Autodesk Inventor part; units mm, degrees
ref_plane "Work Plane1" through (44.45, -80.8985, 0) normal (0, -1, 0) x (1, 0, 0)
ref_plane "YZ Plane" through (0, 0, 0) normal (1, 0, 0) x (0, 1, 0)
ref_plane "XZ Plane" through (0, 0, 0) normal (0, 1, 0) x (-1, 0, 0)
sketch "Sketch1" plane through (0, 0, 0) normal (0, 0, 1) x (1, 0, 0)
  line L0 (0, 0) -> (88.9, 0)
  line L1 (0, 0) -> (-0.8653, 0)
  line L2 (88.9, 0) -> (18.4478, 0)
  line L3 (88.9, 22.8434) -> (88.9, 0)
  line L4 (0, 0) -> (-3, 0)
  line L5 (-3, 0) -> (-3, 76.2)
  line L6 (-3, 76.2) -> (0, 76.2)
  line L7 (0, 76.2) -> (0, 0)
  line L8 (88.9, 0) -> (91.9, 0)
  line L9 (91.9, 0) -> (91.9, 76.2)
  line L10 (91.9, 76.2) -> (88.9, 76.2)
  line L11 (88.9, 76.2) -> (88.9, 0)
  arc A0 (88.9, 76.2) -> (0, 76.2) centre (44.45, 1.8166) ccw
  arc A1 (91.9, 76.2) -> (-3, 76.2) centre (44.45, 4.8166) ccw
  dimension "d8" = 3
  dimension "d9" = 76.2
  dimension "d10" = 88.9
  dimension "d11" = 3
  dimension "d12" = 3
extrude "Extrusion1" add sketch "Sketch1" along normal blind 12.6 contours L1 L4 L5 L6 L7 | L6 A1 L10 A0 | L3 L11 L10 L9 L8
sketch "Sketch2" plane through (91.9, 0, 0) normal (1, 0, 0) x (0, 0, -1)
  line L0 (0, 0) -> (-6.3, 0)
  line L1 (-6.3, 0) -> (-6.3, 30)
  line L2 (-6.3, 30) -> (0, 30)
  line L3 (0, 30) -> (0, 0)
  circle A0 centre (-6.3, 30) radius 2.35
  circle A1 centre (-6.3, 12) radius 2.35
  dimension "d15" = 30
  dimension "d16" = 6.3
  dimension "d17" = 4.7
  dimension "d18" = 4.7
  dimension "d19" = 18
  dimension "d26" = 12
extrude "Extrusion2" cut sketch "Sketch2" against normal through all contours A1 L1 | L1 A1 | A0 L1 L2 | L2 L1 A0
ref_plane "Work Plane1" through (44.45, -80.8985, 0) normal (0, -1, 0) x (1, 0, 0)
sketch "Sketch3" plane through (44.45, -80.8985, 0) normal (0, -1, 0) x (1, 0, 0)
  line L0 (47.45, 0) -> (-47.45, 0)
  line L1 (-47.45, 0) -> (0, 0)
  line L2 (0, 0) -> (0, 6.3)
  line L3 (0, 6.3) -> (-47.45, 6.3)
  line L4 (-47.45, 6.3) -> (-47.45, 0)
  circle A0 centre (0, 6.3) radius 5
  point P0 (-44.45, 0)
  dimension "d22" = 6.3
  dimension "d23" = 10
extrude "Extrusion3" cut sketch "Sketch3" against normal through all contours A0 L3 L2 | L2 L3 A0
properties part number "pulleybracket" material "Iron, Cast"
The model under review builds one solid part; all positions refer to its coordinate system, in mm. A direction names the side the tool comes from. Round coordinates to 2 decimals unless told otherwise and drop trailing zeros. Loops run counter-clockwise (first coordinate to the right, second up) from the corner with the lowest first, then second, coordinate; pieces in that order, holes last. Notation, with made-up numbers: (-2, -37) -> (23, -37) arc R8 ccw to (23, -27) -> close; hole circle Ø3 at (30.25, 16). An arc over 180 degrees is marked (long way). Answer as a JSON object with one key per item and string values. Group by question number.
1) We need section B-B on x = 44.45. Write out the cut boundary in (y, z).
2) We need section C-C on y = 12. Write out the cut boundary in (x, z), then the cut area to 3 significant figures.
3) We need section D-D on z = 6.3. Write out the cut boundary in (x, y).
4) Mouldability with a two-part tool opening along X and no side actions: class faces 1 (the face through (0, 39, 6)), 2 (the face through (47.138, 89.413, 10.516)), 3 (the face through (-3, 38, 6)), 4 (the face through (90, 0, 6)) as released by +X, released by -X, zero draft, split by the parting line, or undercut.
5) For faces 5 (the face through (91.9, 38, 6)), 6 (the face through (88.9, 39, 6)), list the 3-axis set-ups (+Z, -Z, +X, -X, +Y, -Y) from which the entire face can be reached by the end or side of a thin tool; tool diameter is ignored.
6) For line 1 (X direction, y = 52, z = 10); line 2 (Z direction, x = 44, y = 89); line 3 (Z direction, x = 91.05, y = 12), list the stretches that pass through material, from the lowest coordinate up. Write a range as [from, to].
7) We need section A-A on y = 35. Write out the cut boundary in (x, z), then the cut area to 3 significant figures.
Result set:
{
 "1": {"outline": "(88.47, 0) -> (90.53, 0) -> (90.53, 1.3) -> (88.47, 1.3) -> close; (88.47, 11.3) -> (90.53, 11.3) -> (90.53, 12.6) -> (88.47, 12.6) -> close"},
 "2": {"outline": "(-3, 0) -> (0, 0) -> (0, 3.95) -> (-3, 3.95) -> close; (-3, 8.65) -> (0, 8.65) -> (0, 12.6) -> (-3, 12.6) -> close; (88.9, 0) -> (91.9, 0) -> (91.9, 3.95) -> (88.9, 3.95) -> close; (88.9, 8.65) -> (91.9, 8.65) -> (91.9, 12.6) -> (88.9, 12.6) -> close", "area": "47.4 mm²"},
 "3": {"outline": "(-3, 0) -> (0, 0) -> (0, 9.65) -> (-3, 9.65) -> close; (-3, 14.35) -> (0, 14.35) -> (0, 27.65) -> (-3, 27.65) -> close; (-3, 32.35) -> (0, 32.35) -> (0, 76.2) arc R86.65 cw to (39.45, 88.32) -> (39.45, 90.39) arc R85.72 ccw to (-3, 76.2) -> close; (49.45, 88.32) arc R86.65 cw to (88.9, 76.2) -> (88.9, 32.35) -> (91.9, 32.35) -> (91.9, 76.2) arc R85.72 ccw to (49.45, 90.39) -> close; (88.9, 0) -> (91.9, 0) -> (91.9, 9.65) -> (88.9, 9.65) -> close; (88.9, 14.35) -> (91.9, 14.35) -> (91.9, 27.65) -> (88.9, 27.65) -> close"},
 "4": {"face 1": "undercut", "face 2": "undercut", "face 3": "released by -X", "face 4": "zero draft"},
 "5": {"face 5": "+Z, -Z, +X, +Y, -Y", "face 6": "+Z, -Z, -Y"},
 "6": {"line 1": "[-3, 0], [88.9, 91.9]", "line 2": "[0, 1.32], [11.28, 12.6]", "line 3": "[0, 3.95], [8.65, 12.6]"},
 "7": {"outline": "(-3, 0) -> (0, 0) -> (0, 12.6) -> (-3, 12.6) -> close; (88.9, 0) -> (91.9, 0) -> (91.9, 12.6) -> (88.9, 12.6) -> close", "area": "75.6 mm²"}
}
